```python
from build123d import *

# Parameters (mm, degrees)
SKETCH3_W                                       = 57.15
SKETCH3_H                                       = 50
BOSS_EXTRUDE1_DEPTH                             = 8
SKETCH3_3_R                                     = 1.5
SKETCH3_3_R_2                                   = 8
CUT_EXTRUDE2_DEPTH                              = 10
SKETCH4_R                                       = 18.5
CUT_EXTRUDE3_DEPTH                              = 4
BOSS_EXTRUDE2_DEPTH                             = 15
BOSS_EXTRUDE2_DEPTH_BACK                        = 23
SKETCH6_W                                       = 80
SKETCH6_H                                       = 5
CSK_FOR_M3_FLAT_HEAD_MACHINE_SCREW1_D           = 3.4
CSK_FOR_M3_FLAT_HEAD_MACHINE_SCREW1_CSINK_D     = 6.3
CSK_FOR_M3_FLAT_HEAD_MACHINE_SCREW1_CSINK_ANGLE = 90
SKETCH13_R                                      = 6.985
SKETCH13_R_2                                    = 5.08
BOSS_EXTRUDE4_DEPTH                             = 2.54
CUT_EXTRUDE6_REACH                              = 544.7
SKETCH16_R                                      = 1.7
CUT_EXTRUDE7_START                              = -3.175
SKETCH13_2_R                                    = 5.08
CUT_EXTRUDE7_DEPTH                              = 3.175


with BuildPart() as part:
    # Sketch3 → Boss-Extrude1 (new body)
    with BuildSketch(Plane.XY):
        with Locations((0, 25)):
            Rectangle(SKETCH3_W, SKETCH3_H)
    extrude(amount=BOSS_EXTRUDE1_DEPTH)

    # Sketch3<3> → Cut-Extrude2 (cut)
    with BuildSketch(Plane.XY):
        with Locations(Location((-7.75, 38.423393759, 0), (0, 0, 180))):
            Circle(SKETCH3_3_R)
        with Locations(Location((7.75, 38.423393759, 0), (0, 0, 180))):
            Circle(SKETCH3_3_R)
        with Locations(Location((-7.75, 11.576606241, 0), (0, 0, 180))):
            Circle(SKETCH3_3_R)
        with Locations(Location((7.75, 11.576606241, 0), (0, 0, 180))):
            Circle(SKETCH3_3_R)
        with Locations(Location((15.5, 25, 0), (0, 0, 180))):
            Circle(SKETCH3_3_R)
        with Locations(Location((6.062177825, 28.499999999, 0), (0, 0, 180))):
            Circle(SKETCH3_3_R_2)
    extrude(amount=CUT_EXTRUDE2_DEPTH, mode=Mode.SUBTRACT)

    # Sketch4 → Cut-Extrude3 (cut)
    with BuildSketch(Plane.XY.offset(8)):
        with Locations((0, 25)):
            Circle(SKETCH4_R)
    extrude(amount=-CUT_EXTRUDE3_DEPTH, mode=Mode.SUBTRACT)

    # Sketch6 → Boss-Extrude2 (add, two sides: drawn at the far end of the back side and taken through both)
    with BuildSketch(Plane.XY.offset(8).offset(-BOSS_EXTRUDE2_DEPTH_BACK)):
        with Locations((0, 2.5)):
            Rectangle(SKETCH6_W, SKETCH6_H)
    extrude(amount=BOSS_EXTRUDE2_DEPTH + BOSS_EXTRUDE2_DEPTH_BACK)

    # CSK for M3 Flat Head Machine Screw1 (through all)
    with Locations(Plane(origin=(0, 5, 0), x_dir=(1, 0, 0), z_dir=(0, 1, 0))):
        with Locations((-32.5, 7.5), (-32.5, -15.5), (32.5, -15.5), (32.5, 7.5)):
            CounterSinkHole(CSK_FOR_M3_FLAT_HEAD_MACHINE_SCREW1_D / 2, CSK_FOR_M3_FLAT_HEAD_MACHINE_SCREW1_CSINK_D / 2, counter_sink_angle=CSK_FOR_M3_FLAT_HEAD_MACHINE_SCREW1_CSINK_ANGLE)

    # Sketch13 → Boss-Extrude4 (add)
    with BuildSketch(Plane(origin=(0, 0, 0), x_dir=(-1, 0, 0), z_dir=(0, 0, -1))):
        with Locations((20.337822175, 28.499999999)):
            Circle(SKETCH13_R)
        with Locations((20.337822175, 28.499999999)):
            Circle(SKETCH13_R_2, mode=Mode.SUBTRACT)
    extrude(amount=BOSS_EXTRUDE4_DEPTH)

    # Sketch16 → Cut-Extrude6 (cut, up to next)
    with BuildSketch(Plane(origin=(-499.248949842, 16.821159134, -28.308871479), x_dir=(0.05083085086369645, -0.0009181581696577923, 0.9987068546806156), z_dir=(0.03609088653191216, 0.9993480899541042, -0.0009181581696584952)), mode=Mode.PRIVATE) as cut_extrude6_sk1:
        with Locations((44.5, 464.499999998)):
            Circle(SKETCH16_R)
    cut_extrude6_tool1 = extrude(cut_extrude6_sk1.sketch, amount=-CUT_EXTRUDE6_REACH, mode=Mode.PRIVATE) & part.part
    add(cut_extrude6_tool1.solids().sort_by_distance((-33.390455, 0.016084, -7.477347))[0], mode=Mode.SUBTRACT)

    # Sketch13<2> → Cut-Extrude7 (cut)
    with BuildSketch(Plane(origin=(0, 0, 0), x_dir=(-1, 0, 0), z_dir=(0, 0, -1)).offset(CUT_EXTRUDE7_START)):
        with Locations((20.337822175, 28.499999999)):
            Circle(SKETCH13_2_R)
    extrude(amount=CUT_EXTRUDE7_DEPTH, mode=Mode.SUBTRACT)


solid = part.part
```
Geometry: final body of the model. Coordinates: model frame, mm. A direction names the side the tool comes from. Round coordinates to 2 decimals unless told otherwise and drop trailing zeros. Loops run counter-clockwise (first coordinate to the right, second up) from the corner with the lowest first, then second, coordinate; pieces in that order, holes last. Notation, with made-up numbers: (0, 62) -> (57, 62) arc R28 cw to (57, 101) -> close; hole circle Ø6 at (52.5, 83). An arc over 180 degrees is marked (long way). Use one line per item in the form item = value.
Item 1: Cut plane A-A on z = 15.5. Output: boundary loops of the cut face in (x, y), then the cut area to 3 significant figures.
Evaluation:
outline = (-40, 0) -> (-34.2, 0) -> (-34.2, 3.55) -> (-35.65, 5) -> (-40, 5) -> close; (-30.8, 0) -> (30.8, 0) -> (30.8, 3.55) -> (29.35, 5) -> (-29.35, 5) -> (-30.8, 3.55) -> close; (34.2, 0) -> (40, 0) -> (40, 5) -> (35.65, 5) -> (34.2, 3.55) -> close
area = 362 mm2
Item 2: Draft query along Y for faces 1 (the cylindrical face through (16.61, 23.99, 1.97)), 2 (the flat face through (-1, 0, 4)), 3 (the flat face through (0, 50, 4)), 4 (the flat face through (-21, 23, -2.54)). Return one class per face: released by +Y, released by -Y, zero draft, split by the parting line, or undercut.
Evaluation:
face_1 = undercut
face_2 = released by -Y
face_3 = released by +Y
face_4 = zero draft
Item 3: Access query for faces 5 (the flat face through (-28.575, 27, 4)), 6 (the flat face through (28.575, 27, 4)), 7 (the cylindrical face through (-16.307, 25.409, 0.358)). Directions: +Z, -Z, +X, -X, +Y, -Y. A direction counts if a zero-diameter tool reaches every point of the face in a straight line with its end or side. Return the directions, or none.
Evaluation:
face_5 = +Z, -Z, -X, +Y
face_6 = +Z, -Z, +X, +Y
face_7 = -Z
Item 4: Cut plane D-D on y = 28.5. Output: boundary loops of the cut face in (x, z) (3 decimals), then the cut area to 3 significant figures.
Evaluation:
outline = (-28.575, 0) -> (-27.323, 0) -> (-27.323, -2.54) -> (-25.418, -2.54) -> (-25.418, 3.175) -> (-15.258, 3.175) -> (-15.258, -2.54) -> (-13.353, -2.54) -> (-13.353, 0) -> (-1.938, 0) -> (-1.938, 4) -> (-18.166, 4) -> (-18.166, 8) -> (-28.575, 8) -> close; (14.062, 0) -> (28.575, 0) -> (28.575, 8) -> (18.166, 8) -> (18.166, 4) -> (14.062, 4) -> close
area = 225 mm2
Item 5: Material intervals for probe 1 along Z at (x, y) = (-32.5, 1.9); probe 2 along Y at (x, z) = (-7.75, 2.7); probe 3 along Z at (x, y) = (-1.5, 6), sorted ascending.
Evaluation:
probe_1 = -15 to -9.2, -5.8 to 13.8, 17.2 to 23
probe_2 = 0 to 10.08, 13.08 to 36.92, 39.92 to 50
probe_3 = 0 to 8
Item 6: Cut plane C-C on y = 7.5. Output: boundary loops of the cut face in (x, z) (3 decimals).
Evaluation:
outline = (-28.575, 0) -> (28.575, 0) -> (28.575, 8) -> (6, 8) -> (6, 4) -> (-6, 4) -> (-6, 8) -> (-28.575, 8) -> close
Item 7: Contact query for flat-ended pins moving along their axis: pin 1 Ø11.5 at (x, y) = (-20.34, 28.5) entering from -Z; pin 2 Ø12 at (y, z) = (16, -3) entering from +X (3 decimals); pin 3 Ø1.5 at (y, z) = (32, 7) entering from -X (3 decimals). Output: stop coordinate, or through.
Evaluation:
pin_1 = -2.54
pin_2 = 28.575
pin_3 = -28.575
Item 8: Cut plane B-B on x = -8. Output: boundary loops of the cut face in (y, z), then the cut area to 3 significant figures.
Evaluation:
outline = (0, -15) -> (5, -15) -> (5, 0) -> (10.1, 0) -> (10.1, 4) -> (8.32, 4) -> (8.32, 8) -> (5, 8) -> (5, 23) -> (0, 23) -> close; (13.06, 0) -> (36.94, 0) -> (36.94, 4) -> (13.06, 4) -> close; (39.9, 0) -> (50, 0) -> (50, 8) -> (41.68, 8) -> (41.68, 4) -> (39.9, 4) -> close
area = 393 mm2
